Geometry check sheet. Reference: the model listing, model coordinates, mm. A direction names the side the tool comes from. Coordinates: 2 decimals unless noted, no trailing zeros. Order: outer loops, then holes, each group sorted by start corner. A loop starts at its lowest first (then second) coordinate and runs counter-clockwise, first axis right, second up. Notation, with made-up numbers: (84, 63) - (109, 63) arc R13 ccw to (109, 68) - close; hole circle Ø2 at (-20.75, 73). An arc over 180 degrees is marked (long way). One line per item, written item: value. Start each with the question number.
```python
from build123d import *

# Parameters (mm, degrees)
F1_DEPTH = 100


with BuildPart() as f1:
    # F0 (on Front) → F1 (new body)
    with BuildSketch(Plane.XZ):
        with BuildLine():
            Line((0, 15.425), (0, 0))
            Line((0, 0), (15.425, 0))
            Line((15.425, 0), (15.425, 3))
            Line((15.425, 3), (13.36, 3))
            Line((13.36, 3), (13.36, 2))
            Line((13.36, 2), (3.414214, 2))
            Line((3.414214, 2), (11.553662, 10.139449))
            Line((11.553662, 10.139449), (11.553662, 6.139449))
            Line((11.553662, 6.139449), (13.553662, 6.139449))
            Line((13.553662, 6.139449), (13.553662, 12.139449))
            Line((13.553662, 12.139449), (14.414214, 13))
            Line((14.414214, 13), (20, 13))
            Line((20, 13), (20, 16.75))
            ThreePointArc((20, 16.75), (17.701903, 17.701903), (16.75, 20))
            Line((16.75, 20), (13, 20))
            Line((13, 20), (13, 14.414214))
            Line((13, 14.414214), (12.139449, 13.553662))
            Line((12.139449, 13.553662), (6.139449, 13.553662))
            Line((6.139449, 13.553662), (6.139449, 11.553662))
            Line((6.139449, 11.553662), (10.139449, 11.553662))
            Line((10.139449, 11.553662), (2, 3.414214))
            Line((2, 3.414214), (2, 13.36))
            Line((2, 13.36), (3, 13.36))
            Line((3, 13.36), (3, 15.425))
            Line((3, 15.425), (0, 15.425))
        make_face()
    extrude(amount=F1_DEPTH)

    # F2: F1 across face


with BuildPart() as f1_1:
    add(f1.part)
    add(f1.part.mirror(Plane(origin=(20, -50, 14.875), x_dir=(0, 1, 0), z_dir=(1, 0, 0))))

    # F3: F1 across face


with BuildPart() as f1_2:
    add(f1_1.part)
    add(f1_1.part.mirror(Plane(origin=(14.875, -50, 20), x_dir=(1, 0, 0), z_dir=(0, 0, 1))))


solid = f1_2.part
```
Q1. Set-up check for faces 3 (the flat face through (27, -49, 20)), 4 (the flat face through (38, -49, 15.425)): record each of +Z, -Z, +X, -X, +Y, -Y from which the full face is reachable in a straight line by a thin tool's end or side.
Q2. Gauge pin test, flat end, axial feed: P1, Ø3, axis at x = 21.5, y = -60.5, coming from the -Z side. Record the tip position at first contact, or that the pin passes through.
Q3. Cross-section at B-B, the plane x = 31.5. Enter the section's corners in (y, z).
Q4. Material ranges on probe 1 along Z at (x, y) = (14.5, -33.5); probe 2 along Z at (x, y) = (20, -9), recorded low to high.
Q5. Cross-section at A-A, the plane z = 32.5. Enter the section's corners in (x, y), and give its area (3 significant figures).
Q6. Release check for a two-part mould opening along X. For faces 1 (the flat face through (8, -49, 0)), 2 (the flat face through (32, -49, 11.554)) record: released by +X, released by -X, zero draft, split by the parting line, or undercut.
Check result:
1. face 3: +Y, -Y
1. face 4: +X, +Y, -Y
2. P1: stops at z = 13
3. outline: (-100, 0) - (0, 0) - (0, 2) - (-100, 2) - close; (-100, 7.09) - (0, 7.09) - (0, 9.91) - (-100, 9.91) - close; (-100, 11.55) - (0, 11.55) - (0, 13.55) - (-100, 13.55) - close; (-100, 26.45) - (0, 26.45) - (0, 28.45) - (-100, 28.45) - close; (-100, 30.09) - (0, 30.09) - (0, 32.91) - (-100, 32.91) - close; (-100, 38) - (0, 38) - (0, 40) - (-100, 40) - close
4. probe 1: z = 0 to 3, 13 to 27, 37 to 40
4. probe 2: z = 13 to 16.75, 23.25 to 27
5. outline: (0, -100) - (2, -100) - (2, 0) - (0, 0) - close; (6.09, -100) - (8.91, -100) - (8.91, 0) - (6.09, 0) - close; (11.55, -100) - (13.55, -100) - (13.55, 0) - (11.55, 0) - close; (26.45, -100) - (28.45, -100) - (28.45, 0) - (26.45, 0) - close; (31.09, -100) - (33.91, -100) - (33.91, 0) - (31.09, 0) - close; (38, -100) - (40, -100) - (40, 0) - (38, 0) - close
5. area: 1,370 mm2
6. face 1: zero draft
6. face 2: undercut
